Can you work these out from the model? Positions are in its coordinate system, mm. A direction names the side the tool comes from. Round coordinates to 2 decimals unless told otherwise and drop trailing zeros. Loops run counter-clockwise (first coordinate to the right, second up) from the corner with the lowest first, then second, coordinate; pieces in that order, holes last. Notation, with made-up numbers: (11.5, -31) - (56.5, -31) arc R20 cw to (56.5, 1) - close; hole circle Ø10 at (17.25, 16). An arc over 180 degrees is marked (long way). Answer as CSV lines item,"result".
Autodesk Inventor part; units mm, degrees
ref_plane "YZ Plane" through (0, 0, 0) normal (1, 0, 0) x (0, 1, 0)
ref_plane "XZ Plane" through (0, 0, 0) normal (0, 1, 0) x (-1, 0, 0)
ref_plane "XY Plane" through (0, 0, 0) normal (0, 0, 1) x (1, 0, 0)
sketch "Skizze1" plane through (0, 0, 0) normal (0, 0, 1) x (1, 0, 0)
  arc A0 (4.899, 1) -> (-4.899, 1) centre (0, 0) ccw
  line L0 (-17.399, 1) -> (-7.218, 1)
  line L1 (-7.218, 1) -> (-4.899, 1)
  line L2 (4.899, 1) -> (17.399, 1)
  line L3 (17.399, 1) -> (17.399, -3)
  line L4 (-17.399, -3) -> (-17.399, 1)
  arc A1 (4.899, -3) -> (-4.899, -3) centre (0, -4) ccw
  line L5 (17.399, -3) -> (4.899, -3)
  line L6 (-4.899, -3) -> (-17.399, -3)
  dimension "d0" = 10
  dimension "d1" = 1
  dimension "d3" = 10
  dimension "d16" = 4
  dimension "d17" = 12.5
  dimension "d18" = 12.5
extrude "Extrusion1" add sketch "Skizze1" along normal blind 10
fillet "Rundung1" radius 4 2 edges at (-4.899, 1, 5) (4.899, 1, 5)
sketch "Skizze4" plane through (-17.399, 1, 10) normal (0, 1, 0) x (1, 0, 0)
  line L0 (0, 10) -> (9.9157, 10)
  line L1 (0, 10) -> (0, 0)
  line L2 (9.9157, 0) -> (0, 0)
  line L3 (9.9157, 10) -> (9.9157, 0)
  line L4 (34.798, 10) -> (34.798, 0)
  line L5 (24.8823, 10) -> (34.798, 10)
  line L6 (24.8823, 0) -> (24.8823, 10)
  line L7 (34.798, 0) -> (24.8823, 0)
  point P0 (17.399, 10)
  point P1 (4.8401, 5)
  point P2 (29.8401, 5)
  dimension "d19" = 25
hole "Bohrung2" at (-12.5589, 1, 5) at (12.4411, 1, 5) direction (0, -1, 0) diameter 3 end through all
properties part number "Klemme"
Q1. I'm going to push a flat-ended pin straight in: pin 1 Ø1.5 at (x, z) = (-13.5, 7) entering from +Y. Where does the tip first touch, or does it pass through?
Checks:
pin 1,"y = 1"
Q2. If I drill on line 1 along X through (y, z) = (-0.85, 5); line 2 along Y through (x, z) = (14, 5); line 3 along Z through (x, y) = (13.5, -2), over which ranges is the centre line in solid material (lowest first)? Write a range as [from, to].
Checks:
line 1,"[-17.4, -14.06], [-11.06, -3.88], [3.88, 10.94], [13.94, 17.4]"
line 2,"[-3, 1]"
line 3,"[0, 3.94], [6.06, 10]"
Q3. On a 3-axis mill with a long thin cutter (end or side, diameter ignored), from which of +Z, -Z, +X, -X, +Y, -Y can I reach the whole of each face in a straight line? I mean faces 1 (the flat face through (11, 1, 4)), 2 (the flat face through (-11, 1, 4)), 3 (the flat face through (11, -3, 4)). Say none if no direction works.
Checks:
face 1,"+Z, -Z, +X, +Y"
face 2,"+Z, -Z, -X, +Y"
face 3,"+Z, -Z, +X, -X, -Y"
Q4. Imagine slicing it at A-A (y = -0.5). Write out the boundary of the cut face in (x, z), then the cut area to 3 significant figures.
Checks:
outline,"(-17.4, 0) - (-3.57, 0) - (-3.57, 10) - (-17.4, 10) - close; (3.57, 0) - (17.4, 0) - (17.4, 10) - (3.57, 10) - close; hole circle Ø3 at (-12.56, 5); hole circle Ø3 at (12.44, 5)"
area,"262 mm²"
Q5. Imagine slicing it at C-C (x = 3.5). Write out the boundary of the cut face in (y, z).
Checks:
outline,"(-0.43, 0) - (3.57, 0) - (3.57, 10) - (-0.43, 10) - close"
Q6. Imagine slicing it at B-B (z = 5). Count the separate pieces of the cut face and the enclosed holes in it, then the cut area to 3 significant figures.
Checks:
separate pieces,"3"
enclosed holes,"0"
area,"117 mm²"
